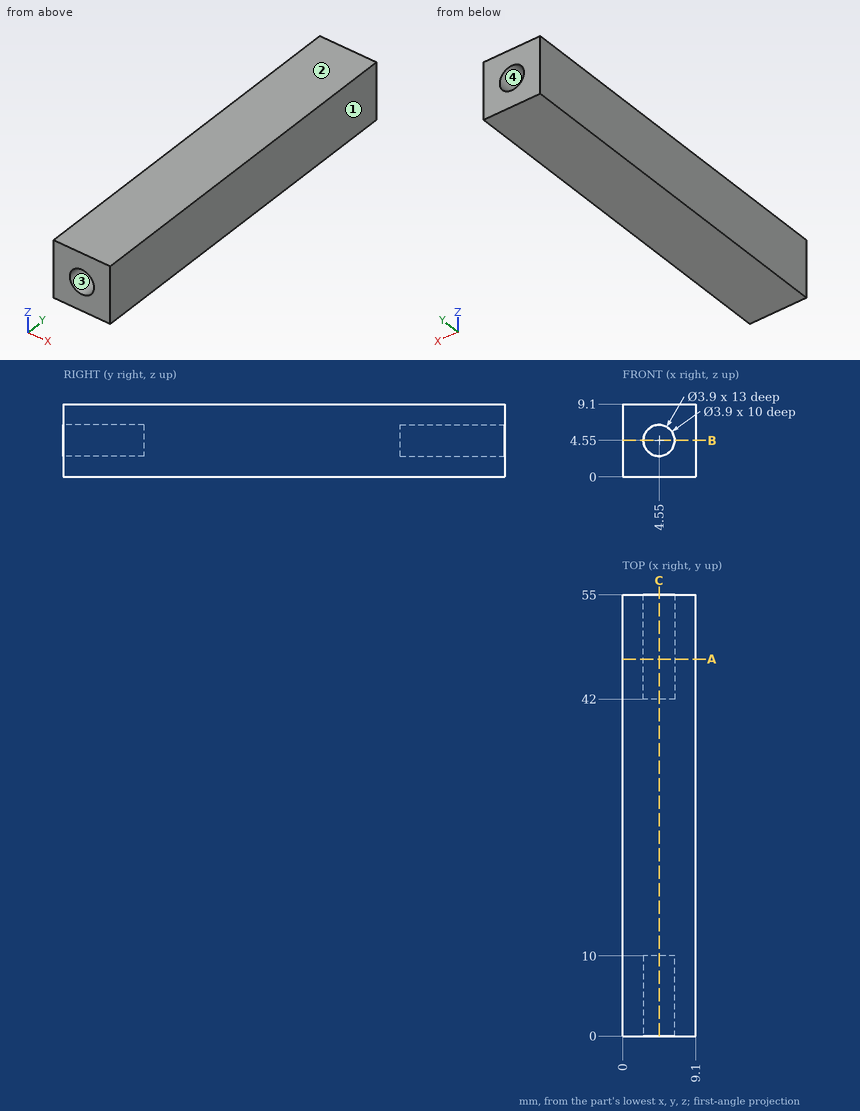
Geometry check sheet. Reference: drawing and pictorial views, mm from the part's lowest x, y, z. Give positions to 0.01 mm unless a question says otherwise; leave off trailing zeros. Write each loop counter-clockwise with the first axis right and the second up, starting at its lowest first coordinate (ties: lowest second). Pieces come first, ordered by that corner, then holes. Notation, with made-up numbers: (25.5, 71) -> (40.5, 71) arc R18 ccw to (40.5, 105) -> close; hole circle Ø7 at (-12.5, 28). An arc over 180 degrees is marked (long way). One line per question, with ' | ' between items.
Item 1: Depth check by flat-ended pin: pin 1 (3 mm diameter, centred on x = 5, z = 5.5, fed in from +Y); pin 2 (1.2 mm diameter, centred on x = 5.5, z = 4.5, fed in from -Y). Enter the tip coordinate at first touch or a pass-through.
Determined:
pin 1: y = 55 | pin 2: y = 10
Item 2: Sectioned sample at A-A, the plane y = 47. Record the boundary of the cut face in (x, z), plus the area to 3 significant figures.
Determined:
outline: (0, 0) -> (9.1, 0) -> (9.1, 9.1) -> (0, 9.1) -> close; hole circle Ø3.9 at (4.55, 4.55) | area: 70.9 mm^2
Item 3: Draft check along Z on the marked faces 1, 2, 3 and 4. Enter one of: released by +Z, released by -Z, zero draft, split by the parting line, or undercut.
Determined:
face 1: zero draft | face 2: released by +Z | face 3: undercut | face 4: undercut
Item 4: Sectioned sample at C-C, the plane x = 4.55. Record the boundary of the cut face in (y, z).
Determined:
outline: (0, 0) -> (55, 0) -> (55, 2.6) -> (42, 2.6) -> (42, 6.5) -> (55, 6.5) -> (55, 9.1) -> (0, 9.1) -> (0, 6.5) -> (10, 6.5) -> (10, 2.6) -> (0, 2.6) -> close
Item 5: Scan lines: line 1 along Z through (x, y) = (4.55, 4.5); line 2 along Y through (x, z) = (5.5, 5.5). Record each from-to range of solid material in increasing order.
Determined:
line 1: 0 to 2.6, 6.5 to 9.1 | line 2: 10 to 42
Item 6: Sectioned sample at B-B, the plane z = 4.55. Record the boundary of the cut face in (x, y).
Determined:
outline: (0, 0) -> (2.6, 0) -> (2.6, 10) -> (6.5, 10) -> (6.5, 0) -> (9.1, 0) -> (9.1, 55) -> (6.5, 55) -> (6.5, 42) -> (2.6, 42) -> (2.6, 55) -> (0, 55) -> close
